For this review, take the finished solid that the model builds, in its own axes (mm). Round coordinates to 2 decimals unless told otherwise and drop trailing zeros. Write each loop counter-clockwise with the first axis right and the second up, starting at its lowest first coordinate (ties: lowest second). Pieces come first, ordered by that corner, then holes. Notation, with made-up numbers: (-5, 84) -> (30, 84) arc R22 ccw to (30, 110) -> close; hole circle Ø11 at (51, 84.5). An arc over 180 degrees is marked (long way). Answer in a Markdown table with one row per item. Add a question column.
```python
from build123d import *

# Parameters (mm, degrees)
SKETCH1_R           = 8
BOSS_EXTRUDE1_DEPTH = 4


with BuildPart() as part:
    # Sketch1 → Boss-Extrude1 (new body)
    with BuildSketch(Plane(origin=(0, 0, 0), x_dir=(1, 0, 0), z_dir=(0, 1, 0))):
        with BuildLine():
            Line((0, 0), (-4, 0))
            ThreePointArc((-4, 0), (-16.7, 12.7), (-29.4, 0))
            Line((-29.4, 0), (-33.4, 0))
            Line((-33.4, 0), (-33.4, 31.8))
            ThreePointArc((-33.4, 31.8), (-16.7, 48.5), (0, 31.8))
            Line((0, 31.8), (0, 0))
        make_face()
        with Locations(Location((-16.7, 31.8, 0), (0, 0, 270))):
            Circle(SKETCH1_R, mode=Mode.SUBTRACT)
    extrude(amount=BOSS_EXTRUDE1_DEPTH)


solid = part.part
```
1. Clearance check with flat-ended pins moving along their axes: pin 1 Ø1 at (x, y) = (-17.5, 3.5) entering from +Z; pin 2 Ø2 at (y, z) = (1, -34.5) entering from -X; pin 3 Ø2 at (y, z) = (2.5, -33) entering from -X. State where each tip first meets the part, or that it passes through.
2. For L1, parallel to X at y = 1.65, z = -31.8; L2, parallel to Z at x = -17, y = 1.4; L3, parallel to Z at x = -11, y = 1.65, list the stretches that pass through material, from the lowest coordinate up. Write a range as [from, to].
3. We need section B-B (y = 3.2). Write out the cut boundary in (x, z).
4. The part is to be moulded in two halves that separate along X. For faces 1 (the cylindrical face through (-16.421, 1.972, -12.697)), 2 (the cylindrical face through (-9.954, 1.972, -27.499)), 3 (the flat face through (-12.8, 4, -24.6)), 4 (the flat face through (-33.4, 2, -16)), say which applies: pulls with the +X half, pulls with the -X half, needs draft (parallel to the pull), parting line crosses it, or undercut.
5. We need section C-C (z = -30). Write out the cut boundary in (x, y).
6. We need section D-D (x = -26). Write out the cut boundary in (y, z), plus the area to 3 significant figures.
7. We need section A-A (x = -16.7). Write out the cut boundary in (y, z).
Response:
| question | item | result |
|---|---|---|
| 1 | pin 1 | z = -12.63 |
| 1 | pin 2 | x = -33.31 |
| 1 | pin 3 | x = -33.4 |
| 2 | L1 | [-33.4, -24.7], [-8.7, 0] |
| 2 | L2 | [-48.5, -39.79], [-23.81, -12.7] |
| 2 | L3 | [-47.5, -37.41], [-26.19, -11.35] |
| 3 | outline | (-33.4, -31.8) arc R16.7 ccw to (0, -31.8) -> (0, 0) -> (-4, 0) arc R12.7 cw to (-29.4, 0) -> (-33.4, 0) -> close; hole circle Ø16 at (-16.7, -31.8) |
| 4 | face 1 | undercut |
| 4 | face 2 | undercut |
| 4 | face 3 | needs draft |
| 4 | face 4 | pulls with the -X half |
| 5 | outline | (-33.4, 0) -> (-24.49, 0) -> (-24.49, 4) -> (-33.4, 4) -> close; (-8.91, 0) -> (0, 0) -> (0, 4) -> (-8.91, 4) -> close |
| 6 | outline | (0, -45.67) -> (4, -45.67) -> (4, -8.65) -> (0, -8.65) -> close |
| 6 | area | 148 mm2 |
| 7 | outline | (0, -48.5) -> (4, -48.5) -> (4, -39.8) -> (0, -39.8) -> close; (0, -23.8) -> (4, -23.8) -> (4, -12.7) -> (0, -12.7) -> close |
